The model under review builds one solid part; all positions refer to its coordinate system, in mm. Face numbers are marked on the shaded views. A direction names the side the tool comes from. Coordinates: 2 decimals unless noted, no trailing zeros. Loops run counter-clockwise (first coordinate to the right, second up) from the corner with the lowest first, then second, coordinate; pieces in that order, holes last. Notation, with made-up numbers: (16.5, 77.25) -> (47.5, 77.25) arc R25 cw to (47.5, 95.25) -> close; hole circle Ø2 at (51, -6). An arc over 180 degrees is marked (long way). One line per question, with ' | ' between items. Start each with the question number.
from build123d import *

# Parameters (mm, degrees)
SKETCH1_W           = 240
SKETCH1_H           = 80
SKETCH1_W_2         = 180
SKETCH1_H_2         = 30
BOSS_EXTRUDE1_DEPTH = 5
SKETCH2_W           = 5
SKETCH2_H           = 80
BOSS_EXTRUDE2_DEPTH = 20
SKETCH4_W           = 5
SKETCH4_H           = 80
BOSS_EXTRUDE3_DEPTH = 20
SKETCH3_R           = 3
CUT_EXTRUDE1_DEPTH  = 245.591496173


with BuildPart() as part:
    # Sketch1 → Boss-Extrude1 (new body)
    with BuildSketch(Plane(origin=(0, 0, 0), x_dir=(1, 0, 0), z_dir=(0, 1, 0))):
        Rectangle(SKETCH1_W, SKETCH1_H)
        Rectangle(SKETCH1_W_2, SKETCH1_H_2, mode=Mode.SUBTRACT)
    extrude(amount=BOSS_EXTRUDE1_DEPTH)

    # Sketch2 → Boss-Extrude2 (add)
    with BuildSketch(Plane(origin=(0, 5, 0), x_dir=(1, 0, 0), z_dir=(0, 1, 0))):
        with Locations((117.5, 0)):
            Rectangle(SKETCH2_W, SKETCH2_H)
    extrude(amount=BOSS_EXTRUDE2_DEPTH)

    # Sketch4 → Boss-Extrude3 (add)
    with BuildSketch(Plane(origin=(0, 5, 0), x_dir=(1, 0, 0), z_dir=(0, 1, 0))):
        with Locations((-117.5, 0)):
            Rectangle(SKETCH4_W, SKETCH4_H)
    extrude(amount=BOSS_EXTRUDE3_DEPTH)

    # Sketch3 → Cut-Extrude1 (cut, through all)
    with BuildSketch(Plane(origin=(120, 0, 0), x_dir=(0, 0, -1), z_dir=(1, 0, 0))):
        with Locations((-25, 15)):
            Circle(SKETCH3_R)
        with Locations(Location((25, 15, 0), (0, 0, 180))):
            Circle(SKETCH3_R)
    extrude(amount=-CUT_EXTRUDE1_DEPTH, mode=Mode.SUBTRACT)


solid = part.part
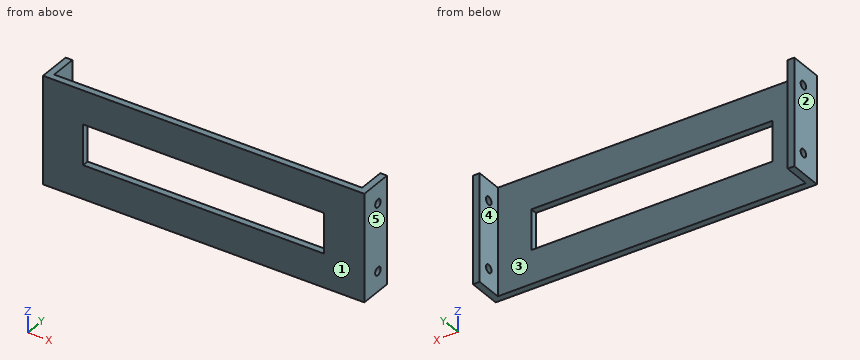
1) Consider section B-B, the plane z = -5.5. Write out the cut boundary in (x, y), plus the area to 3 significant figures.
2) Wall thickness on L1, parallel to X at y = 15.75, z = 36.5; L2, parallel to Y at x = -118.45, z = 25; L3, parallel to Z at x = -86, y = 2: over which ranges is each line inside the solid? List them lowest first.
3) Mouldability with a two-part tool opening along X and no side actions: class the marked faces 1, 2 and 3 as +X half, -X half, draft (parallel to the pull), parting line (faces both ways), or undercut.
4) Consider section D-D, the plane y = 2.75. Write out the cut boundary in (x, z), plus the area to 3 significant figures.
5) Consider section C-C, the plane x = -53.5. Write out the cut boundary in (y, z), plus the area to 3 significant figures.
6) Insertion check: pin 1 Ø2 at (x, z) = (25.5, -26.5) entering from +Y. The pin has a flat end and moves straight along its axis. Give the tip position at first contact, or say it passes through.
7) Consider section A-A, the plane y = 21. Write out the cut boundary in (x, z).
8) Machinability: for the marked faces 4 and 5, which of the approach directions +Z, -Z, +X, -X, +Y, -Y give a long, thin tool a straight path to every point of the face, cutting with its end or side? Answer none if there is none.
Filled sheet:
1) outline: (-120, 0) -> (-90, 0) -> (-90, 5) -> (-115, 5) -> (-115, 25) -> (-120, 25) -> close; (90, 0) -> (120, 0) -> (120, 25) -> (115, 25) -> (115, 5) -> (90, 5) -> close | area: 500 mm^2
2) L1: -120 to -115, 115 to 120 | L2: 0 to 12, 18 to 25 | L3: -40 to -15, 15 to 40
3) face 1: draft | face 2: -X half | face 3: undercut
4) outline: (-120, -40) -> (120, -40) -> (120, 40) -> (-120, 40) -> close; hole (-90, -15) -> (90, -15) -> (90, 15) -> (-90, 15) -> close | area: 13,800 mm^2
5) outline: (0, -40) -> (5, -40) -> (5, -15) -> (0, -15) -> close; (0, 15) -> (5, 15) -> (5, 40) -> (0, 40) -> close | area: 250 mm^2
6) pin 1: y = 5
7) outline: (-120, -40) -> (-115, -40) -> (-115, 40) -> (-120, 40) -> close; (115, -40) -> (120, -40) -> (120, 40) -> (115, 40) -> close
8) face 4: +Z, -Z, +Y | face 5: +Z, -Z, +X, +Y, -Y
